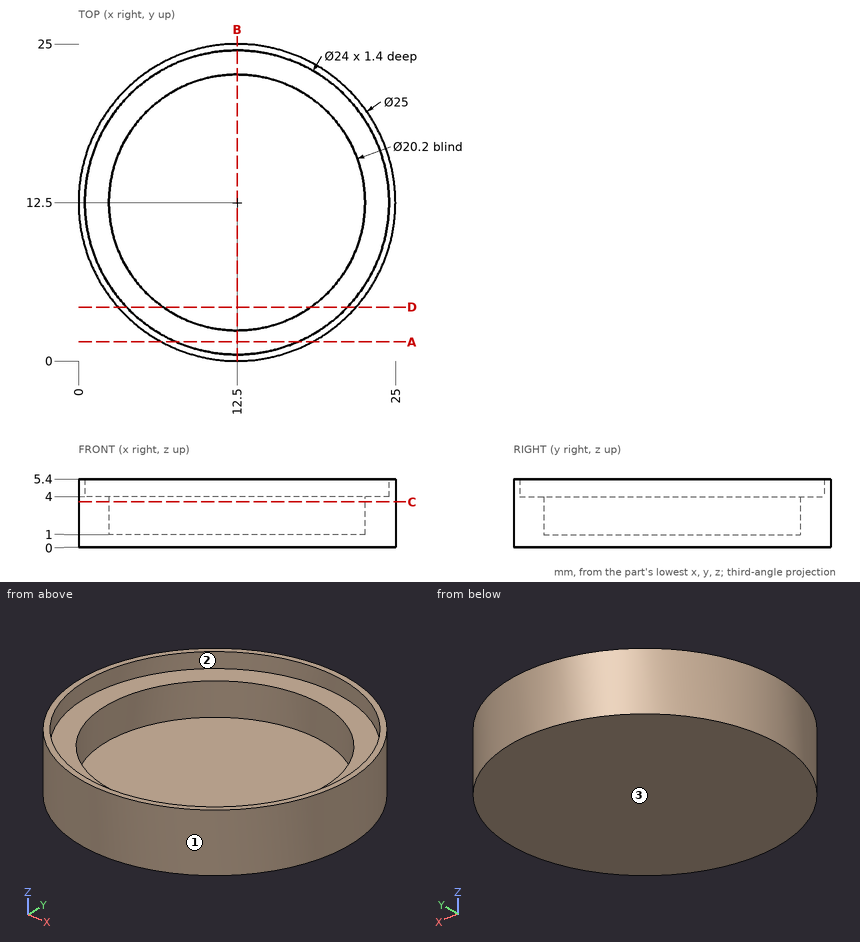
Check sheet for the drawn part. Datum: minimum x, y, z corner. Units: mm. Give positions to 0.01 mm unless a question says otherwise; leave off trailing zeros. Loops run counter-clockwise (first coordinate to the right, second up) from the corner with the lowest first, then second, coordinate; pieces in that order, holes last.
1) Thickness scan on line 1 along Y through (x, z) = (12.5, 2.55); line 2 along Z through (x, y) = (12.5, 2); line 3 along Y through (x, z) = (9, 4.7). Record the ranges inside material, lowest first.
2) Sectioned sample at C-C, the plane z = 3.6. Enter the section's corners in (x, y).
3) Sectioned sample at B-B, the plane x = 12.5. Enter the section's corners in (y, z).
4) Draft check along X on the marked faces 1, 2 and 3. Enter one of: pulls with the +X half, pulls with the -X half, needs draft (parallel to the pull), parting line crosses it, or undercut.
5) Sectioned sample at A-A, the plane y = 1.5. Enter the section's corners in (x, z).
6) Sectioned sample at D-D, the plane y = 4.25. Enter the section's corners in (x, z), then the cut area to 3 significant figures.
7) Depth check by flat-ended pin: pin 1 Ø2 at (y, z) = (14.5, 4) entering from +X; pin 2 Ø10 at (x, y) = (17.5, 16) entering from +Z. Enter the tip coordinate at first touch or a pass-through.
Answers:
1. line 1: y = 0 to 2.4, 22.6 to 25
1. line 2: z = 0 to 4
1. line 3: y = 0.5 to 1.02, 23.98 to 24.5
2. outline: circle Ø25 at (12.5, 12.5); hole circle Ø20.2 at (12.5, 12.5)
3. outline: (0, 0) - (25, 0) - (25, 5.4) - (24.5, 5.4) - (24.5, 4) - (22.6, 4) - (22.6, 1) - (2.4, 1) - (2.4, 4) - (0.5, 4) - (0.5, 5.4) - (0, 5.4) - close
4. face 1: parting line crosses it
4. face 2: undercut
4. face 3: needs draft
5. outline: (6.56, 0) - (18.44, 0) - (18.44, 5.4) - (17.3, 5.4) - (17.3, 4) - (7.7, 4) - (7.7, 5.4) - (6.56, 5.4) - close
6. outline: (3.11, 0) - (21.89, 0) - (21.89, 5.4) - (21.21, 5.4) - (21.21, 4) - (18.33, 4) - (18.33, 1) - (6.67, 1) - (6.67, 4) - (3.79, 4) - (3.79, 5.4) - (3.11, 5.4) - close
6. area: 42.1 mm2
7. pin 1: stops at x = 24.96
7. pin 2: stops at z = 4
